from build123d import *

# Parameters (mm, degrees)
CYLINDER004_R           = 9.5
CYLINDER004_DEPTH       = 25
CYLINDER004_PITCH_ANGLE = 90
CYLINDER003_R           = 11
CYLINDER003_DEPTH       = 105
CYLINDER003_PITCH_ANGLE = 90
CYLINDER002_R           = 12.5
CYLINDER002_DEPTH       = 130
CYLINDER002_PITCH_ANGLE = 90


with BuildPart() as cylinder002:
    # Cylinder004 → Cylinder004 (new body)
    with BuildSketch(Plane.XY):
        Circle(CYLINDER004_R)
    extrude(amount=CYLINDER004_DEPTH)


with BuildPart() as cylinder002_1:
    # Cylinder004 pitch: moved
    add(cylinder002.part.rotate(Axis((0, 0, 0), (0, 1, 0)), CYLINDER004_PITCH_ANGLE))


with BuildPart() as cylinder002_2:
    # Cylinder004 placement: moved
    add(cylinder002_1.part.moved(Location((156, 0, 0))))


with BuildPart() as cylinder001:
    # Cylinder003 → Cylinder003 (new body)
    with BuildSketch(Plane.XY):
        Circle(CYLINDER003_R)
    extrude(amount=CYLINDER003_DEPTH)


with BuildPart() as cylinder001_1:
    # Cylinder003 pitch: moved
    add(cylinder001.part.rotate(Axis((0, 0, 0), (0, 1, 0)), CYLINDER003_PITCH_ANGLE))


with BuildPart() as cylinder001_2:
    # Cylinder003 placement: moved
    add(cylinder001_1.part.moved(Location((51, 0, 0))))


with BuildPart() as batteryholder:
    # Cylinder002 → Cylinder002 (new body)
    with BuildSketch(Plane.XY):
        Circle(CYLINDER002_R)
    extrude(amount=CYLINDER002_DEPTH)


with BuildPart() as batteryholder_1:
    # Cylinder002 pitch: moved
    add(batteryholder.part.rotate(Axis((0, 0, 0), (0, 1, 0)), CYLINDER002_PITCH_ANGLE))


with BuildPart() as batteryholder_2:
    # Cylinder002 placement: moved
    add(batteryholder_1.part.moved(Location((51, 0, 0))))

    # Cut001: cut Cylinder001
    add(cylinder001_2.part, mode=Mode.SUBTRACT)

    # Cut002: cut Cylinder002
    add(cylinder002_2.part, mode=Mode.SUBTRACT)


solid = batteryholder_2.part
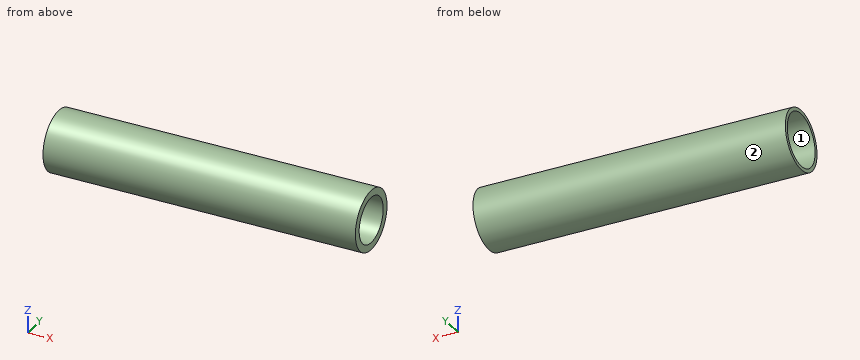
Part model, mm, in its own coordinate system. Face numbers are marked on the shaded views. Give positions to 0.01 mm unless a question says otherwise; leave off trailing zeros. Loops run counter-clockwise (first coordinate to the right, second up) from the corner with the lowest first, then second, coordinate; pieces in that order, holes last. Notation, with made-up numbers: (13, -26) -> (66, -26) arc R33 ccw to (66, 11) -> close; hole circle Ø11 at (36.25, 62). An arc over 180 degrees is marked (long way). Write each question's results on one line, items separated by ' | '. Start each with the question number.
Q1. Pull direction Z, two halves, no side cores. Call the marked faces 1 and 2: +Z half, -Z half, draft (parallel to the pull), parting line (faces both ways), or undercut.
Q2. Band-saw the part on C-C on x = 68. List the corners of the cut face in (y, z).
Q3. Pin check, flat tips, straight feed: P1, Ø6, axis at x = 161, z = -6.5, coming from the +Y side; P2, Ø1.5, axis at x = 141, y = -5, coming from the -Z side; P3, Ø4, axis at x = 65, z = -3, coming from the -Y side; P4, Ø13, axis at y = 0, z = 0, coming from the +X side. Stop position of each tip, or through.
Q4. Wall check: L1, parallel to Y at x = 85.5, z = 0; L2, parallel to X at y = -1.25, z = -10.5; L3, parallel to Z at x = 107.5, y = -1.5. Give the ranges that are in metal, low to high.
Q5. Band-saw the part on A-A on y = 0. List the corners of the cut face in (x, z), plus the area to 3 significant figures.
Results are:
1) face 1: undercut | face 2: parting line
2) outline: circle Ø25 at (0, 0); hole circle Ø22 at (0, 0)
3) P1: stops at y = 12 | P2: stops at z = -11.76 | P3: stops at y = -12.46 | P4: passes through
4) L1: y = -12.5 to -11, 11 to 12.5 | L2: x = 156 to 181 | L3: z = -12.41 to -10.9, 10.9 to 12.41
5) outline: (51, -12.5) -> (181, -12.5) -> (181, -9.5) -> (156, -9.5) -> (156, -11) -> (51, -11) -> close; (51, 11) -> (156, 11) -> (156, 9.5) -> (181, 9.5) -> (181, 12.5) -> (51, 12.5) -> close | area: 465 mm²
